Geometry: final body of the model. Coordinates: model frame, mm. A direction names the side the tool comes from. Coordinates: 2 decimals unless noted, no trailing zeros. Write each loop counter-clockwise with the first axis right and the second up, starting at its lowest first coordinate (ties: lowest second). Pieces come first, ordered by that corner, then holes. Notation, with made-up numbers: M 73.5,83 L 78.5,83 A23 ccw 78.5,100 Z; hole C 25,-36 d2. An arc over 180 degrees is marked long. Write item = value, one per line. Start each with the question number.
Item 1: Section A-A on x = -6.5. Output: boundary loops of the cut face in (y, z).
Item 2: Ray query, L1, parallel to Y at x = 0, z = 3.8; L2, parallel to Y at x = 18, z = 1.85; L3, parallel to X at y = 9, z = 2.5. Return the intervals inside material, ascending. Write a range as [from, to].
Item 3: Reachability of faces 1 (the flat face through (-15.31, -11.56, 2.71)), 2 (the flat face through (-17.67, 7.48, 2.71)), 3 (the flat face through (20.167, -4.121, 2.712)), 4 (the flat face through (19.525, 6.514, 2.712)), 5 (the flat face through (15.31, 11.56, 2.71)) from +Z, -Z, +X, -X, +Y, -Y: full face, straight path, thin tool, end or side. Return the list, or none.
Item 4: Pull-direction query (X, two-part tool) for faces 6 (the cylindrical face through (-6.468, -4.959, 2.788)), 7 (the flat face through (11.56, -15.31, 2.71)), 8 (the flat face through (7.48, 17.67, 2.71)), 9 (the flat face through (-15.428, -13.626, 2.712)); classes: +X half, -X half, draft (parallel to the pull), parting line (faces both ways), or undercut.
Item 5: First-contact query: pin 1 Ø2 at (y, z) = (13, 1.5) entering from -X; pin 2 Ø1 at (y, z) = (-16.5, 4.5) entering from -X. Flat tips, straight axial feed; report the tip coordinate or a pass-through.
from build123d import *

# Parameters (mm, degrees)
ROLLER_SEATING_TOOTH_PROFILE_DEPTH = 5.5
SKETCH_2_R                         = 8.15
THROUGH_SHAFT_BORE_DEPTH           = 30.398963933


with BuildPart() as part:
    # 草图1 → Roller_seating_tooth_profile (new body)
    with BuildSketch(Plane.XY):
        Polygon((19.919196173, -5.337332529), (20.421178717, -2.870009502), (17.706188737, -1.860995427), (17.217421057, -1.203959364), (16.990472298, -0.593320367), (16.921869331, 0), (16.990472298, 0.593320367), (17.217421057, 1.203959364), (17.706188737, 1.860995427), (20.421178717, 2.870009502), (19.919196173, 5.337332529), (19.120264295, 7.72508822), (16.264506963, 7.241425053), (15.512703705, 7.566051134), (15.010840815, 7.981405639), (14.65476872, 8.460934666), (14.417520449, 9.009066659), (14.308744341, 9.651369923), (14.403511537, 10.464763684), (16.250254793, 12.696090496), (14.581863645, 14.581863645), (12.696090496, 16.250254793), (10.464763684, 14.403511537), (9.651369923, 14.308744341), (9.009066659, 14.417520449), (8.460934666, 14.65476872), (7.981405639, 15.010840815), (7.566051134, 15.512703705), (7.241425053, 16.264506963), (7.72508822, 19.120264295), (5.337332529, 19.919196173), (2.870009502, 20.421178717), (1.860995427, 17.706188737), (1.203959364, 17.217421057), (0.593320367, 16.990472298), (0, 16.921869331), (-0.593320367, 16.990472298), (-1.203959364, 17.217421057), (-1.860995427, 17.706188737), (-2.870009502, 20.421178717), (-5.337332529, 19.919196173), (-7.72508822, 19.120264295), (-7.241425053, 16.264506963), (-7.566051134, 15.512703705), (-7.981405639, 15.010840815), (-8.460934666, 14.65476872), (-9.009066659, 14.417520449), (-9.651369923, 14.308744341), (-10.464763684, 14.403511537), (-12.696090496, 16.250254793), (-14.581863645, 14.581863645), (-16.250254793, 12.696090496), (-14.403511537, 10.464763684), (-14.308744341, 9.651369923), (-14.417520449, 9.009066659), (-14.65476872, 8.460934666), (-15.010840815, 7.981405639), (-15.512703705, 7.566051134), (-16.264506963, 7.241425053), (-19.120264295, 7.72508822), (-19.919196173, 5.337332529), (-20.421178717, 2.870009502), (-17.706188737, 1.860995427), (-17.217421057, 1.203959364), (-16.990472298, 0.593320367), (-16.921869331, 0), (-16.990472298, -0.593320367), (-17.217421057, -1.203959364), (-17.706188737, -1.860995427), (-20.421178717, -2.870009502), (-19.919196173, -5.337332529), (-19.120264295, -7.72508822), (-16.264506963, -7.241425053), (-15.512703705, -7.566051134), (-15.010840815, -7.981405639), (-14.65476872, -8.460934666), (-14.417520449, -9.009066659), (-14.308744341, -9.651369923), (-14.403511537, -10.464763684), (-16.250254793, -12.696090496), (-14.581863645, -14.581863645), (-12.696090496, -16.250254793), (-10.464763684, -14.403511537), (-9.651369923, -14.308744341), (-9.009066659, -14.417520449), (-8.460934666, -14.65476872), (-7.981405639, -15.010840815), (-7.566051134, -15.512703705), (-7.241425053, -16.264506963), (-7.72508822, -19.120264295), (-5.337332529, -19.919196173), (-2.870009502, -20.421178717), (-1.860995427, -17.706188737), (-1.203959364, -17.217421057), (-0.593320367, -16.990472298), (0, -16.921869331), (0.593320367, -16.990472298), (1.203959364, -17.217421057), (1.860995427, -17.706188737), (2.870009502, -20.421178717), (5.337332529, -19.919196173), (7.72508822, -19.120264295), (7.241425053, -16.264506963), (7.566051134, -15.512703705), (7.981405639, -15.010840815), (8.460934666, -14.65476872), (9.009066659, -14.417520449), (9.651369923, -14.308744341), (10.464763684, -14.403511537), (12.696090496, -16.250254793), (14.581863645, -14.581863645), (16.250254793, -12.696090496), (14.403511537, -10.464763684), (14.308744341, -9.651369923), (14.417520449, -9.009066659), (14.65476872, -8.460934666), (15.010840815, -7.981405639), (15.512703705, -7.566051134), (16.264506963, -7.241425053), (19.120264295, -7.72508822), align=None)
    extrude(amount=ROLLER_SEATING_TOOTH_PROFILE_DEPTH)

    # 草图2 → Through_shaft_bore (cut, through all)
    with BuildSketch(Plane.XY.offset(5.5)):
        Circle(SKETCH_2_R)
    extrude(amount=-THROUGH_SHAFT_BORE_DEPTH, mode=Mode.SUBTRACT)


solid = part.part
Responses:
q1.outline = M -19.53,0 L -4.92,0 L -4.92,5.5 L -19.53,5.5 Z; M 4.92,0 L 19.53,0 L 19.53,5.5 L 4.92,5.5 Z
q2.L1 = [-16.92, -8.15], [8.15, 16.92]
q2.L2 = [-7.54, -1.97], [1.97, 7.54]
q2.L3 = [-14.42, 14.42]
q3.face_1 = +Z, -Z, -X
q3.face_2 = +Z, -Z, +Y
q3.face_3 = +Z, -Z, +X, -Y
q3.face_4 = +Z, -Z, +X, +Y
q3.face_5 = +Z, -Z, +X
q4.face_6 = undercut
q4.face_7 = undercut
q4.face_8 = +X half
q4.face_9 = -X half
q5.pin_1 = -16.25
q5.pin_2 = -12.98
